```python
from build123d import *

# Parameters (mm, degrees)
SKETCH1_W                  = 39.999999999
SKETCH1_H                  = 30
BOSS_EXTRUDE1_DEPTH        = 3.175
SKETCH3_W                  = 3.175
SKETCH3_H                  = 3.175
SKETCH3_W_2                = 25
BOSS_EXTRUDE2_DEPTH        = 40
SKETCH4_R                  = 2.5
CUT_EXTRUDE1_DEPTH         = 10
FILLET1_R                  = 7
CONVERT_SOLID1_START       = -32.140684808
CONVERT_SOLID1_OUTLINE_R   = 2.5
CONVERT_SOLID1_DEPTH       = 5.340684808
CONVERT_SOLID1_START_2     = -33.2
CONVERT_SOLID1_2_OUTLINE_R = 2.5
CONVERT_SOLID1_2_DEPTH     = 0.025
CONVERT_SOLID1_START_3     = -27.475968
CONVERT_SOLID1_3_OUTLINE_W = 39.999999999
CONVERT_SOLID1_3_OUTLINE_H = 0.025
CONVERT_SOLID1_3_DEPTH     = 27.475968
CONVERT_SOLID1_START_4     = 31.592932584
CONVERT_SOLID1_4_DEPTH     = 39.999999999
CONVERT_SOLID1_START_5     = -49
CONVERT_SOLID1_5_OUTLINE_W = 39.999999999
CONVERT_SOLID1_5_OUTLINE_H = 3.2
CONVERT_SOLID1_5_DEPTH     = 2.85856
CONVERT_SOLID1_START_6     = 3.175
CONVERT_SOLID1_6_DEPTH     = 0.825


with BuildPart() as part:
    # Sketch1 → Boss-Extrude1 (new body)
    with BuildSketch(Plane.XY):
        with Locations((51.592932584, -15)):
            Rectangle(SKETCH1_W, SKETCH1_H)
        with BuildLine():
            Line((34.092932584, -11.25), (34.092932584, -7.25))
            ThreePointArc((34.092932584, -7.25), (36.592932584, -4.75), (39.092932584, -7.25))
            Line((39.092932584, -7.25), (39.092932584, -11.25))
            ThreePointArc((39.092932584, -11.25), (36.592932584, -13.75), (34.092932584, -11.25))
        make_face(mode=Mode.SUBTRACT)
        with BuildLine():
            Line((64.092932583, -11.25), (64.092932583, -7.25))
            ThreePointArc((64.092932583, -7.25), (66.592932583, -4.75), (69.092932583, -7.25))
            Line((69.092932583, -7.25), (69.092932583, -11.25))
            ThreePointArc((69.092932583, -11.25), (66.592932583, -13.75), (64.092932583, -11.25))
        make_face(mode=Mode.SUBTRACT)
    extrude(amount=BOSS_EXTRUDE1_DEPTH)


with BuildPart() as body_2:
    # Mirror1: mirrored copy
    add(part.part.mirror(Plane(origin=(0, -15, -15), x_dir=(0, -0.7071067811865465, 0.7071067811865486), z_dir=(0, -0.7071067811865488, -0.7071067811865464))))


with BuildPart() as part_1:
    add(part.part)

    add(body_2.part)  # Boss-Extrude2 merges body 2
    # Sketch3 → Boss-Extrude2 (add, through all)
    with BuildSketch(Plane(origin=(71.592932583, 0, 0), x_dir=(0, 0, -1), z_dir=(1, 0, 0))):
        with Locations((-1.5875, -31.5875)):
            Rectangle(SKETCH3_W, SKETCH3_H)
        with Locations((42.5, -31.5875)):
            Rectangle(SKETCH3_W_2, SKETCH3_H)
    extrude(amount=-BOSS_EXTRUDE2_DEPTH)

    # Sketch4 → Cut-Extrude1 (cut)
    with BuildSketch(Plane.XZ.offset(33.175)):
        with Locations((61.592932583, -45)):
            Circle(SKETCH4_R)
        with Locations((41.592932584, -45)):
            Circle(SKETCH4_R)
    extrude(amount=-CUT_EXTRUDE1_DEPTH, mode=Mode.SUBTRACT)

    # Fillet1
    fillet1_edges = [part_1.edges().sort_by_distance(p)[0] for p in [
        (31.592932584, 0, 1.5875),
        (71.592932583, 0, 1.5875),
        (71.592932583, -31.5875, -55),
        (31.592932583, -31.5875, -55),
    ]]
    fillet(fillet1_edges, radius=FILLET1_R)

    # Convert-Solid1: read off the stored shape, not the designer's step
    # Convert-Solid1 outline → Convert-Solid1 (add)
    with BuildSketch(Plane(origin=(0, 0, 0), x_dir=(1, 0, 0), z_dir=(0, 1, 0)).offset(CONVERT_SOLID1_START)):
        with BuildLine():
            Line((31.592932584, 48), (31.592932584, 0))
            Line((31.592932584, 0), (71.592932583, 0))
            Line((71.592932583, 0), (71.592932583, 48))
            ThreePointArc((71.592932583, 48), (69.542680051, 52.949747468), (64.592932583, 55))
            Line((64.592932583, 55), (38.592932584, 55))
            ThreePointArc((38.592932584, 55), (33.643185116, 52.949747469), (31.592932584, 48))
        make_face()
        with BuildLine():
            ThreePointArc((34.092932584, 22.75), (36.592932584, 25.25), (39.092932584, 22.75))
            Line((39.092932584, 22.75), (39.092932584, 18.75))
            ThreePointArc((39.092932584, 18.75), (36.592932584, 16.25), (34.092932584, 18.75))
            Line((34.092932584, 18.75), (34.092932584, 22.75))
        make_face(mode=Mode.SUBTRACT)
        with BuildLine():
            ThreePointArc((64.092932583, 22.75), (66.592932583, 25.25), (69.092932583, 22.75))
            Line((69.092932583, 22.75), (69.092932583, 18.75))
            ThreePointArc((69.092932583, 18.75), (66.592932583, 16.25), (64.092932583, 18.75))
            Line((64.092932583, 18.75), (64.092932583, 22.75))
        make_face(mode=Mode.SUBTRACT)
        with Locations((41.592932584, 45)):
            Circle(CONVERT_SOLID1_OUTLINE_R, mode=Mode.SUBTRACT)
        with Locations((61.592932583, 45)):
            Circle(CONVERT_SOLID1_OUTLINE_R, mode=Mode.SUBTRACT)
    extrude(amount=CONVERT_SOLID1_DEPTH)

    # Convert-Solid1 2 outline → Convert-Solid1 2 (add)
    with BuildSketch(Plane(origin=(0, 0, 0), x_dir=(1, 0, 0), z_dir=(0, 1, 0)).offset(CONVERT_SOLID1_START_2)):
        with BuildLine():
            Line((31.592932584, 48), (31.592932584, 0))
            Line((31.592932584, 0), (71.592932583, 0))
            Line((71.592932583, 0), (71.592932583, 48))
            ThreePointArc((71.592932583, 48), (69.542680051, 52.949747468), (64.592932583, 55))
            Line((64.592932583, 55), (38.592932584, 55))
            ThreePointArc((38.592932584, 55), (33.643185116, 52.949747469), (31.592932584, 48))
        make_face()
        with BuildLine():
            ThreePointArc((34.092932584, 22.75), (36.592932584, 25.25), (39.092932584, 22.75))
            Line((39.092932584, 22.75), (39.092932584, 18.75))
            ThreePointArc((39.092932584, 18.75), (36.592932584, 16.25), (34.092932584, 18.75))
            Line((34.092932584, 18.75), (34.092932584, 22.75))
        make_face(mode=Mode.SUBTRACT)
        with BuildLine():
            ThreePointArc((64.092932583, 22.75), (66.592932583, 25.25), (69.092932583, 22.75))
            Line((69.092932583, 22.75), (69.092932583, 18.75))
            ThreePointArc((69.092932583, 18.75), (66.592932583, 16.25), (64.092932583, 18.75))
            Line((64.092932583, 18.75), (64.092932583, 22.75))
        make_face(mode=Mode.SUBTRACT)
        with Locations((41.592932584, 45)):
            Circle(CONVERT_SOLID1_2_OUTLINE_R, mode=Mode.SUBTRACT)
        with Locations((61.592932583, 45)):
            Circle(CONVERT_SOLID1_2_OUTLINE_R, mode=Mode.SUBTRACT)
    extrude(amount=CONVERT_SOLID1_2_DEPTH)

    # Convert-Solid1 3 outline → Convert-Solid1 3 (add)
    with BuildSketch(Plane(origin=(0, 0, 0), x_dir=(1, 0, 0), z_dir=(0, 1, 0)).offset(CONVERT_SOLID1_START_3)):
        with Locations((51.592932584, -3.1875)):
            Rectangle(CONVERT_SOLID1_3_OUTLINE_W, CONVERT_SOLID1_3_OUTLINE_H)
    extrude(amount=CONVERT_SOLID1_3_DEPTH)

    # Convert-Solid1 4 outline → Convert-Solid1 4 (cut)
    with BuildSketch(Plane.YZ.offset(CONVERT_SOLID1_START_4)):
        with BuildLine():
            ThreePointArc((-26.8, 0), (-29.0627417, -0.9372583), (-30, -3.2))
            Line((-30, -3.2), (-30, -55))
            Line((-30, -55), (-26.8, -55))
            Line((-26.8, -55), (-26.8, 0))
        make_face()
        with BuildLine():
            Line((-33.2, 0), (-33.2, -3.2))
            ThreePointArc((-33.2, -3.2), (-31.3254834, 1.3254834), (-26.8, 3.2))
            Line((-26.8, 3.2), (-27.475968, 3.2))
            Line((-27.475968, 3.2), (-27.475968, 3.175))
            Line((-27.475968, 3.175), (-33.175, 3.175))
            Line((-33.175, 3.175), (-33.175, 0))
            Line((-33.175, 0), (-33.2, 0))
        make_face()
    extrude(amount=CONVERT_SOLID1_4_DEPTH, mode=Mode.SUBTRACT)

    # Convert-Solid1 5 outline → Convert-Solid1 5 (cut)
    with BuildSketch(Plane.XY.offset(CONVERT_SOLID1_START_5)):
        with Locations((51.592932584, -28.4)):
            Rectangle(CONVERT_SOLID1_5_OUTLINE_W, CONVERT_SOLID1_5_OUTLINE_H)
    extrude(amount=CONVERT_SOLID1_5_DEPTH, mode=Mode.SUBTRACT)

    # Convert-Solid1 6 outline → Convert-Solid1 6 (cut)
    with BuildSketch(Plane.XY.offset(CONVERT_SOLID1_START_6)):
        with BuildLine():
            Line((71.592932583, -7), (71.592932583, 0))
            Line((71.592932583, 0), (64.592932583, 0))
            ThreePointArc((64.592932583, 0), (69.542680051, -2.050252532), (71.592932583, -7))
        make_face()
        with BuildLine():
            ThreePointArc((31.592932584, -7), (33.643185116, -2.050252531), (38.592932584, 0))
            Line((38.592932584, 0), (31.592932584, 0))
            Line((31.592932584, 0), (31.592932584, -7))
        make_face()
        with BuildLine():
            ThreePointArc((64.092932583, -11.25), (66.592932583, -13.75), (69.092932583, -11.25))
            Line((69.092932583, -11.25), (69.092932583, -7.25))
            ThreePointArc((69.092932583, -7.25), (66.592932583, -4.75), (64.092932583, -7.25))
            Line((64.092932583, -7.25), (64.092932583, -11.25))
        make_face()
        with BuildLine():
            ThreePointArc((34.092932584, -11.25), (36.592932584, -13.75), (39.092932584, -11.25))
            Line((39.092932584, -11.25), (39.092932584, -7.25))
            ThreePointArc((39.092932584, -7.25), (36.592932584, -4.75), (34.092932584, -7.25))
            Line((34.092932584, -7.25), (34.092932584, -11.25))
        make_face()
    extrude(amount=CONVERT_SOLID1_6_DEPTH, mode=Mode.SUBTRACT)


solid = part_1.part
```
Verification items for the finished model (mm, model axes). A direction names the side the tool comes from. Round coordinates to 2 decimals unless told otherwise and drop trailing zeros. Write each loop counter-clockwise with the first axis right and the second up, starting at its lowest first coordinate (ties: lowest second). Pieces come first, ordered by that corner, then holes. Notation, with made-up numbers: (-39.75, 57) - (14.25, 57) arc R22 cw to (14.25, 84) - close; hole circle Ø7 at (22, 59). An arc over 180 degrees is marked (long way). Answer as a JSON object with one key per item and string values. Group by question number.
Q1. Go/stop test with flat-tipped pins: pin 1 Ø8 at (x, z) = (61.59, -45) entering from -Y; pin 2 Ø6 at (x, z) = (41.59, -45) entering from +Y; pin 3 Ø12 at (x, y) = (43.5, -23) entering from -Z; pin 4 Ø2 at (x, y) = (43.5, -7.5) entering from -Z. Record where each tip stops, or that it passes through.
Q2. Section check C-C, the plane x = 41. Enter the section's corners in (y, z).
Q3. Section check B-B, the plane y = -8.5. Enter the section's corners in (x, z).
Q4. Section check A-A, the plane x = 67. Enter the section's corners in (y, z) (3 decimals).
Q5. Tool access check on faces 1 (the flat face through (51, -13, 0)), 2 (the flat face through (51, 0, 2)), 3 (the flat face through (34.093, -9, 2)), 4 (the cylindrical face through (66.65, -31.62, -16.25)). Record the directions out of +Z, -Z, +X, -X, +Y, -Y that give a thin tool (end or side, any length) a straight path to the whole face; none if there is none.
Q6. Mould release check, pull along X, two halves, no side actions. Record for faces 5 (the cylindrical face through (43.9, -31.62, -45.96)), 6 (the flat face through (71.593, -31, -11)), 7 (the flat face through (39.093, -32, -21)), 8 (the cylindrical face through (51.31, -31.37, 1.28)): released by +X, released by -X, zero draft, split by the parting line, or undercut.
Q7. Section check D-D, the plane x = 50.5. Enter the section's corners in (y, z).
Q8. Thickness scan on line 1 (X direction, y = -32, z = -45); line 2 (X direction, y = -30.5, z = -21.5); line 3 (Y direction, x = 56.5, z = -48). Record the ranges inside material, lowest first.
Found:
{
 "1": {"pin 1": "stops at y = -33.2", "pin 2": "stops at y = -30", "pin 3": "stops at z = -0.88", "pin 4": "stops at z = 0"},
 "2": {"outline": "(-33.2, -55) - (-30, -55) - (-30, -47.43) - (-33.2, -47.43) - close; (-33.2, -42.57) - (-30, -42.57) - (-30, -3.2) arc R3.2 cw to (-26.8, 0) - (0, 0) - (0, 3.2) - (-26.8, 3.2) arc R6.4 ccw to (-33.2, -3.2) - close"},
 "3": {"outline": "(31.59, 0) - (34.09, 0) - (34.09, 3.2) - (31.59, 3.2) - close; (39.09, 0) - (64.09, 0) - (64.09, 3.2) - (39.09, 3.2) - close; (69.09, 0) - (71.59, 0) - (71.59, 3.2) - (69.09, 3.2) - close"},
 "4": {"outline": "(-33.2, -54.573) - (-30, -54.573) - (-30, -25.217) - (-33.2, -25.217) - close; (-33.2, -16.283) - (-30, -16.283) - (-30, -3.2) arc R3.2 cw to (-26.8, 0) - (-13.717, 0) - (-13.717, 3.2) - (-26.8, 3.2) arc R6.4 ccw to (-33.2, -3.2) - close; (-4.783, 0) - (-0.427, 0) - (-0.427, 3.2) - (-4.783, 3.2) - close"},
 "5": {"face 1": "-Z, +X, -X, +Y", "face 2": "+Z, -Z, +X, -X, +Y", "face 3": "+Z, -Z", "face 4": "+Y, -Y"},
 "6": {"face 5": "undercut", "face 6": "released by +X", "face 7": "undercut", "face 8": "zero draft"},
 "7": {"outline": "(-33.2, -55) - (-30, -55) - (-30, -3.2) arc R3.2 cw to (-26.8, 0) - (0, 0) - (0, 3.2) - (-26.8, 3.2) arc R6.4 ccw to (-33.2, -3.2) - close"},
 "8": {"line 1": "x = 31.59 to 39.09, 44.09 to 59.09, 64.09 to 71.59", "line 2": "x = 31.59 to 34.09, 39.09 to 64.09, 69.09 to 71.59", "line 3": "y = -33.2 to -30"}
}
